from build123d import *

# Parameters (mm, degrees)
SKETCH_1_W          = 55
SKETCH_1_H          = 8
EXTRUDE_1_DEPTH     = 5
SKETCH_2_W          = 4.8
SKETCH_2_H          = 2
CUT_EXTRUDE_1_DEPTH = 9
CHAMFER_1_SIZE      = 1.5


with BuildPart() as part:
    # 草图1 → 凸台-拉伸1 (new body)
    with BuildSketch(Plane(origin=(0, 0, 0), x_dir=(1, 0, 0), z_dir=(0, 1, 0))):
        Rectangle(SKETCH_1_W, SKETCH_1_H)
    extrude(amount=EXTRUDE_1_DEPTH)

    # 草图2 → 切除-拉伸1 (cut, through all)
    with BuildSketch(Plane.XY.offset(4)):
        with Locations((-19.6, 4)):
            Rectangle(SKETCH_2_W, SKETCH_2_H)
        with Locations((-9.8, 4)):
            Rectangle(SKETCH_2_W, SKETCH_2_H)
        with Locations((0, 4)):
            Rectangle(SKETCH_2_W, SKETCH_2_H)
        with Locations((9.8, 4)):
            Rectangle(SKETCH_2_W, SKETCH_2_H)
        with Locations((19.6, 4)):
            Rectangle(SKETCH_2_W, SKETCH_2_H)
    extrude(amount=-CUT_EXTRUDE_1_DEPTH, mode=Mode.SUBTRACT)

    # 倒角1
    chamfer_1_edges = [part.edges().sort_by_distance(p)[0] for p in [
        (-27.5, 5, 0),
        (-27.5, 0, 0),
    ]]
    chamfer(chamfer_1_edges, length=CHAMFER_1_SIZE)


solid = part.part
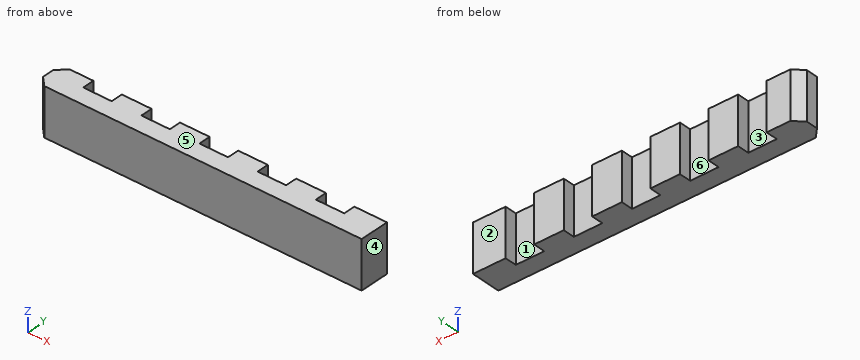
Read the model definition and answer for the solid it produces. Units are mm, in the model's axes. Face numbers are marked on the shaded views. A direction names the side the tool comes from. Round coordinates to 2 decimals unless told otherwise and drop trailing zeros. Order: outer loops, then holes, each group sorted by start corner. A loop starts at its lowest first (then second) coordinate and runs counter-clockwise, first axis right, second up. Notation, with made-up numbers: (76, -35) - (111, -35) arc R21 cw to (111, -17) - close; hole circle Ø5 at (78.25, -22.5). An arc over 180 degrees is marked (long way). Use one line per item in the form item = value. Start each with the question number.
(1) The part is cut by section A-A (y = 4.35). Give the vertices of the cut face in (x, z), then the cut area to 3 significant figures.
(2) Flat-ended cylindrical pins translate along their axes: pin 1 Ø1.4 at (x, z) = (-19, 0.5) entering from +Y; pin 2 Ø1 at (y, z) = (4.5, 1) entering from -X; pin 3 Ø0.6 at (y, z) = (4.5, -2) entering from -X. Find the tip coordinate at first contact, or state that the pin passes through.
(3) Find the intervals of material crossed by line 1 along X through (y, z) = (3.5, 0); line 2 along X through (y, z) = (3.7, -3.5); line 3 along Y through (x, z) = (1.5, -2.25), in increasing order. Write a range as from..to.
(4) For the marked faces 5 and 6, determine the directions among +Z, -Z, +X, -X, +Y, -Y from which every point of the face is accessible in a straight line to the end or side of a thin tool.
(5) Determine the mould class of the marked faces 1, 2, 3 and 4 for opening direction X: +X half, -X half, draft (parallel to the pull), parting line (faces both ways), or undercut.
(6) The part is cut by section B-B (z = -2.5). Give the vertices of the cut face in (x, y).
(7) The part is cut by section C-C (y = 0.65). Give the vertices of the cut face in (x, z).
Checked values:
q1.outline = (-26.65, -4) - (-22, -4) - (-22, 4) - (-26.65, 4) - close; (-17.2, -4) - (-12.2, -4) - (-12.2, 4) - (-17.2, 4) - close; (-7.4, -4) - (-2.4, -4) - (-2.4, 4) - (-7.4, 4) - close; (2.4, -4) - (7.4, -4) - (7.4, 4) - (2.4, 4) - close; (12.2, -4) - (17.2, -4) - (17.2, 4) - (12.2, 4) - close; (22, -4) - (27.5, -4) - (27.5, 4) - (22, 4) - close
q1.area = 241 mm^2
q2.pin_1 = 3
q2.pin_2 = -27
q2.pin_3 = -26.8
q3.line_1 = -27.5..-22, -17.2..-12.2, -7.4..-2.4, 2.4..7.4, 12.2..17.2, 22..27.5
q3.line_2 = -27.3..-22, -17.2..-12.2, -7.4..-2.4, 2.4..7.4, 12.2..17.2, 22..27.5
q3.line_3 = 0..3
q4.face_5 = +Z, +X, -X, +Y, -Y
q4.face_6 = +Z, -Z, +Y
q5.face_1 = undercut
q5.face_2 = draft
q5.face_3 = undercut
q5.face_4 = +X half
q6.outline = (-27.5, 1.5) - (-26, 0) - (27.5, 0) - (27.5, 5) - (22, 5) - (22, 3) - (17.2, 3) - (17.2, 5) - (12.2, 5) - (12.2, 3) - (7.4, 3) - (7.4, 5) - (2.4, 5) - (2.4, 3) - (-2.4, 3) - (-2.4, 5) - (-7.4, 5) - (-7.4, 3) - (-12.2, 3) - (-12.2, 5) - (-17.2, 5) - (-17.2, 3) - (-22, 3) - (-22, 5) - (-26, 5) - (-27.5, 3.5) - close
q7.outline = (-26.65, -4) - (27.5, -4) - (27.5, 4) - (-26.65, 4) - close
